Design review of the part built by this model. Coordinates are the model's own, in mm. A direction names the side the tool comes from. Coordinates: 2 decimals unless noted, no trailing zeros. Loops run counter-clockwise (first coordinate to the right, second up) from the corner with the lowest first, then second, coordinate; pieces in that order, holes last. Notation, with made-up numbers: (8.25, 34) - (29.25, 34) arc R5 ccw to (29.25, 38) - close; hole circle Ø10 at (33.5, 67.25). An arc over 180 degrees is marked (long way). One line per question, with ' | ' between items.
Autodesk Inventor part; units mm, degrees
ref_plane "YZ Plane" through (0, 0, 0) normal (1, 0, 0) x (0, 1, 0)
ref_plane "XZ Plane" through (0, 0, 0) normal (0, 1, 0) x (-1, 0, 0)
ref_plane "XY Plane" through (0, 0, 0) normal (0, 0, 1) x (1, 0, 0)
sketch "Sketch1" plane through (0, 0, 0) normal (0, 0, 1) x (1, 0, 0)
  circle A0 centre (0, 0) radius 3.9624
  dimension "d0" = 7.9248
extrude "Extrusion1" add sketch "Sketch1" along normal blind 4.826
sketch "Sketch2" plane through (0, 0, 0) normal (0, 0, -1) x (-1, 0, 0)
  circle A0 centre (0, 0) radius 3.9624
  circle A1 centre (0, 0) radius 2.413
  dimension "d3" = 4.826
extrude "Extrusion2" add sketch "Sketch2" along normal blind 69.85 contours A1
sketch "Sketch3" plane through (0, 0, 4.826) normal (0, 0, 1) x (1, 0, 0)
  circle A0 centre (0, 0) radius 3.9624
  line L0 (-1.1457, 1.9844) -> (1.1457, 1.9844)
  line L1 (1.1457, 1.9844) -> (2.2914, 0)
  line L2 (2.2914, 0) -> (1.1457, -1.9844)
  line L3 (1.1457, -1.9844) -> (-1.1457, -1.9844)
  line L4 (-1.1457, -1.9844) -> (-2.2914, 0)
  line L5 (-2.2914, 0) -> (-1.1457, 1.9844)
  dimension "d6" = 3.9688
extrude "Extrusion3" cut sketch "Sketch3" against normal blind 3.175 contours L0 L1 L2 L3 L4 L5
thread "Thread1"
chamfer "Chamfer1" distance 0.508 angle 45 1 edges at (2.413, 0, -69.85)
chamfer "Chamfer2" distance 0.508 angle 45 1 edges at (-3.9624, 0, 4.826)
properties part number "10-32 x1000" material "Steel"
Q1. Take a section at A-A (x = 0). Give the boundary of the cut face in (y, z) (3 decimals), plus the area to 3 significant figures.
Returned:
outline: (-3.962, 0) - (-2.413, 0) - (-2.413, -69.342) - (-1.905, -69.85) - (1.905, -69.85) - (2.413, -69.342) - (2.413, 0) - (3.962, 0) - (3.962, 4.318) - (3.454, 4.826) - (1.984, 4.826) - (1.984, 1.651) - (-1.984, 1.651) - (-1.984, 4.826) - (-3.454, 4.826) - (-3.962, 4.318) - close | area: 362 mm²
Q2. To check wall thickness, follow line 1 along Y through (x, z) = (-0.25, -21); line 2 along Y through (x, z) = (-1.5, -29); line 3 along Z through (x, y) = (-1, -1.25). State the ranges of each line that lie inside material, in increasing order.
Returned:
line 1: y = -2.4 to 2.4 | line 2: y = -1.89 to 1.89 | line 3: z = -69.85 to 1.65
Q3. Draft analysis for pull direction Y (two halves, no side actions). For faces 1 (the flat face through (-1.727, 0.978, 3.261)), 2 (the cylindrical face through (-0.52, -3.93, 2.13)), 3 (the flat face through (-2, -1, 4.826)), state which applies: +Y half, -Y half, draft (parallel to the pull), parting line (faces both ways), or undercut.
Returned:
face 1: undercut | face 2: parting line | face 3: draft
Q4. Tool access review of faces 4 (the flat face through (2, 2, 0)), 5 (the flat face through (-1.71, -1.01, 3.26)), 6 (the flat face through (0, 0, -69.85)): name each direction out of +Z, -Z, +X, -X, +Y, -Y from which nothing blocks a thin tool from reaching the whole face with its end or side.
Returned:
face 4: -Z | face 5: +Z | face 6: -Z, +X, -X, +Y, -Y
Q5. For pin 1 (2 mm diameter, centred on x = -0.5, z = -16, fed in from -Y); pin 2 (3 mm diameter, centred on y = 1, z = -53, fed in from +X); pin 3 (3 mm diameter, centred on x = 2, z = -25.5, fed in from +Y); pin 4 (3 mm diameter, centred on x = -1, y = 0.5, fed in from +Z), all flat-tipped, find the tip position at first contact; note any pin that passes through.
Returned:
pin 1: stops at y = -2.41 | pin 2: stops at x = 2.41 | pin 3: stops at y = 2.36 | pin 4: stops at z = 4.83
Q6. Take a section at B-B (z = -18). Give the boundary of the cut face in (x, y), plus the area to 3 significant figures.
Returned:
outline: circle Ø4.83 at (0, 0) | area: 18.3 mm²
